```python
from build123d import *

# Parameters (mm, degrees)
F0_W      = 15
F0_H      = 3
F1_DEPTH  = 15
F2_DEPTH  = 3
F3_DEPTH  = 3
F4_DEPTH  = 2
F5_DEPTH  = 3
F6_DEPTH  = 12
F7_D      = 5
F7_DEPTH  = 15
F7_TIP    = 1.5021515476
F9_W      = 3.15
F9_H      = 15
F10_DEPTH = 17
F11_R     = 1
F12_W     = 50
F12_H     = 100
F13_DEPTH = 5
F14_R     = 4.99999


# Not quite as in the source:
# - a fillet or chamfer is up to 0.001 mm smaller than in the source, because OpenCascade refuses the exact size


with BuildPart() as f1:
    # F0 (on Right) → F1 (new body)
    with BuildSketch(Plane.YZ):
        with Locations((0, 1.5)):
            Rectangle(F0_W, F0_H)
    extrude(amount=-F1_DEPTH)

    # F0 (on Right) → F2 (join)
    with BuildSketch(Plane.YZ):
        with BuildLine():
            Line((-7.5, 12.5), (-7.5, 3))
            Line((-7.5, 3), (7.5, 3))
            Line((7.5, 3), (7.5, 12.5))
            ThreePointArc((7.5, 12.5), (0, 20), (-7.5, 12.5))
        make_face()
        Polygon((-6.25, 12.5), (-3.125, 17.9126587737), (3.125, 17.9126587737), (6.25, 12.5), (3.125, 7.0873412263), (-3.125, 7.0873412263), align=None, mode=Mode.SUBTRACT)
    extrude(amount=-F2_DEPTH)

    # F0 (on Right) → F3 (join)
    with BuildSketch(Plane.YZ):
        Polygon((3.125, 17.9126587737), (-3.125, 17.9126587737), (-6.25, 12.5), (-3.125, 7.0873412263), (3.125, 7.0873412263), (6.25, 12.5), align=None)
        Polygon((-4.9074772881, 12.5), (-2.4537386441, 16.75), (2.4537386441, 16.75), (4.9074772881, 12.5), (2.4537386441, 8.25), (-2.4537386441, 8.25), align=None, mode=Mode.SUBTRACT)
    extrude(amount=-F3_DEPTH)

    # F0 (on Right) → F4 (join)
    with BuildSketch(Plane.YZ):
        Polygon((3.125, 17.9126587737), (-3.125, 17.9126587737), (-6.25, 12.5), (-3.125, 7.0873412263), (3.125, 7.0873412263), (6.25, 12.5), align=None)
        Polygon((-4.9074772881, 12.5), (-2.4537386441, 16.75), (2.4537386441, 16.75), (4.9074772881, 12.5), (2.4537386441, 8.25), (-2.4537386441, 8.25), align=None, mode=Mode.SUBTRACT)
    extrude(amount=F4_DEPTH)

    # F0 (on Right) → F5 (join)
    with BuildSketch(Plane.YZ):
        Polygon((2.4537386441, 16.75), (-2.4537386441, 16.75), (-4.9074772881, 12.5), (-2.4537386441, 8.25), (2.4537386441, 8.25), (4.9074772881, 12.5), align=None)
    extrude(amount=-F5_DEPTH)

    # F6 (add): a face of the model
    f6_faces = [f1.faces().sort_by_distance(p)[0] for p in [
        (-3, 0, 10.7862789639),
    ]]
    extrude(f6_faces, amount=F6_DEPTH)

    # F7
    with Locations(Plane.YZ):
        with Locations((0, 12.5)):
            Hole(F7_D / 2, depth=F7_DEPTH)
            with Locations((0, 0, -(F7_DEPTH + F7_TIP / 2))):  # 118° drill point
                Cone(0, F7_D / 2, F7_TIP, mode=Mode.SUBTRACT)

    # F9 (on offset) → F10 (cut)
    with BuildSketch(Plane.XY.offset(20)):
        with Locations((-10.475, 0)):
            Rectangle(F9_W, F9_H)
        with Locations((-4.525, 0)):
            Rectangle(F9_W, F9_H)
    extrude(amount=-F10_DEPTH, mode=Mode.SUBTRACT)

    # F11
    f11_edges = [f1.edges().sort_by_distance(p)[0] for p in [
        (2, -4.6875, 9.793671),
        (2, 0, 7.087341),
        (2, -4.6875, 15.206329),
        (2, 0, 17.912659),
        (2, 4.6875, 15.206329),
        (2, 4.6875, 9.793671),
    ]]
    fillet(f11_edges, radius=F11_R)

    # F12 (on Top) → F13 (join)
    with BuildSketch(Plane.XY):
        with Locations((-5.9974378107, 0)):
            Rectangle(F12_W, F12_H)
    extrude(amount=-F13_DEPTH)

    # F14 (radius 5 in the source; OpenCascade refuses exactly that, so slightly less here)
    f14_edges = [f1.edges().sort_by_distance(p)[0] for p in [
        (-5.997438, 50, 0),
        (19.002562, 0, 0),
        (-5.997438, -50, 0),
        (-30.997438, 0, 0),
    ]]
    fillet(f14_edges, radius=F14_R)


solid = f1.part
```
Geometry: final body of the model. Coordinates: model frame, mm. A direction names the side the tool comes from. Round coordinates to 2 decimals unless told otherwise and drop trailing zeros. Order: outer loops, then holes, each group sorted by start corner. A loop starts at its lowest first (then second) coordinate and runs counter-clockwise, first axis right, second up. Notation, with made-up numbers: M 26.5,41 L 58.5,41 A22 ccw 58.5,74 Z; hole C 57,-29.75 d4. An arc over 180 degrees is marked long. Use one line per item in the form item = value. Start each with the question number.
Q1. Material intervals for line 1 (X direction, y = 2.5, z = 10); line 2 (Z direction, x = -7.05, y = 0); line 3 (X direction, y = 3, z = 7.75), sorted ascending. Write a range as [from, to].
Q2. Cut plane A-A (z = 4.25). Return loops of the section in (x, y).
Q3. Mould query, pull axis Z, two halves, no side actions, for faces 6 (the face through (0, 0, 6)), 7 (the face through (1.715, -4.449, 15.018)), 8 (the face through (-2.95, -0.1, 9.7)). Classes: +Z half, -Z half, draft (parallel to the pull), parting line (faces both ways), or undercut.
Q4. Access query for faces 1 (the face through (-7, 7.5, 5)), 2 (the face through (0.49, -4.71, 9.83)), 3 (the face through (-5, 0, 3)), 4 (the face through (0, 2.1, 10.7)), 5 (the face through (1.715, 4.449, 9.982)). Directions: +Z, -Z, +X, -X, +Y, -Y. A direction counts if a zero-diameter tool reaches every point of the face in a straight line with its end or side. Return the directions, or none.
Q5. Cut plane D-D (y = 0). Count the separate pieces of the cut face and the enclosed holes in it, and give its area (3 significant figures).
Q6. Pin query (flat end, axial travel): pin 1 Ø0.5 at (x, y) = (0.5, 1) entering from +Z; pin 2 Ø4 at (x, z) = (-6.5, 6) entering from -Y; pin 3 Ø1.6 at (x, y) = (-11, -1.5) entering from +Z. Return the tip coordinate at first contact, or that it passes through.
Geometry results:
q1.line_1 = [-15, -12.05], [-8.9, -6.1], [-2.95, 0]
q1.line_2 = [-5, 10], [15, 20]
q1.line_3 = [-15, -12.05], [-8.9, -6.1], [-2.95, 1.83]
q2.outline = M -15,-7.5 L -12.05,-7.5 L -12.05,7.5 L -15,7.5 Z; M -8.9,-7.5 L -6.1,-7.5 L -6.1,7.5 L -8.9,7.5 Z; M -2.95,-7.5 L 0,-7.5 L 0,7.5 L -2.95,7.5 Z
q3.face_6 = undercut
q3.face_7 = +Z half
q3.face_8 = draft
q4.face_1 = +Z, +X, -X, +Y
q4.face_2 = +X, -Y
q4.face_3 = +Z, +Y, -Y
q4.face_4 = +X
q4.face_5 = +X, +Y
q5.separate_pieces = 4
q5.enclosed_holes = 0
q5.area = 393 mm^2
q6.pin_1 = 17.91
q6.pin_2 = -7.5
q6.pin_3 = 3
